Geometry: final body of the model. Coordinates: model frame, mm. Give positions to 0.01 mm unless a question says otherwise; leave off trailing zeros. Write each loop counter-clockwise with the first axis right and the second up, starting at its lowest first coordinate (ties: lowest second). Pieces come first, ordered by that corner, then holes. Notation, with made-up numbers: (26.25, 88.25) - (40.25, 88.25) arc R30 ccw to (40.25, 124.25) - close; hole circle Ø7 at (-33.75, 30). An arc over 180 degrees is marked (long way). Return JSON: item names as keys, results as strings.
from build123d import *

# Parameters (mm, degrees)
SKETCH1_W          = 20
SKETCH1_H          = 3
SKETCH1_R          = 0.5
BASE_FLANGE1_DEPTH = 0.7366


# Sheet-metal steps are written as plain solids
with BuildPart() as part:
    # Sketch1 → Base-Flange1 (new body)
    with BuildSketch(Plane(origin=(0, 0, 0), x_dir=(1, 0, 0), z_dir=(0, 1, 0))):
        Rectangle(SKETCH1_W, SKETCH1_H)
        with Locations(Location((-9, 0, 0), (0, 0, 270))):
            Circle(SKETCH1_R, mode=Mode.SUBTRACT)
    extrude(amount=-BASE_FLANGE1_DEPTH)


solid = part.part
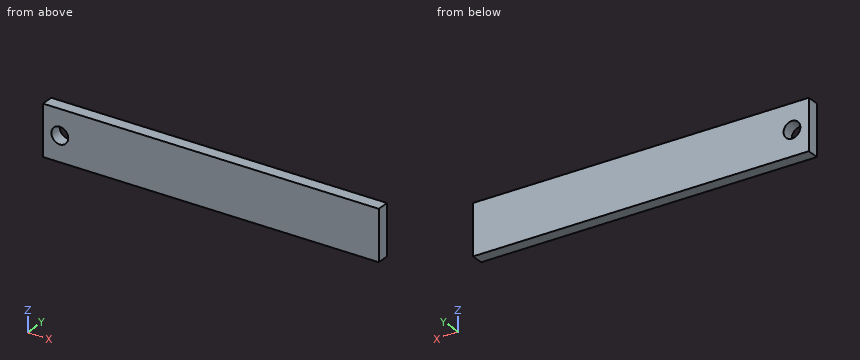
Q1. Material intervals for probe 1 along X at (y, z) = (-0.3, 0); probe 2 along X at (y, z) = (-0.05, -0.3), sorted ascending. Write a range as [from, to].
Answer key:
{"probe 1": "x = [-10, -9.5], [-8.5, 10]", "probe 2": "x = [-10, -9.4], [-8.6, 10]"}
Q2. Section query B-B, the plane z = 0. Return the cut outline in (x, y).
Answer key:
{"outline": "(-10, -0.74) - (-9.5, -0.74) - (-9.5, 0) - (-10, 0) - close; (-8.5, -0.74) - (10, -0.74) - (10, 0) - (-8.5, 0) - close"}
Q3. Section query A-A, the plane x = -9. Return the cut outline in (y, z), plus the area to 3 significant figures.
Answer key:
{"outline": "(-0.74, -1.5) - (0, -1.5) - (0, -0.5) - (-0.74, -0.5) - close; (-0.74, 0.5) - (0, 0.5) - (0, 1.5) - (-0.74, 1.5) - close", "area": "1.47 mm^2"}
